Geometry: see drawing. Coordinates: mm, zero at the bounding-box minimum. A direction names the side the tool comes from. Coordinates: 2 decimals unless noted, no trailing zeros. Loops run counter-clockwise (first coordinate to the right, second up) from the corner with the lowest first, then second, coordinate; pieces in that order, holes last. Notation, with made-up numbers: (37.5, 20) -> (71.5, 20) arc R29 ccw to (71.5, 44) -> close; hole circle Ø3 at (86.25, -22). An arc over 180 degrees is marked (long way). Put each result on its own line as item: value. Start each with the question number.
1) Contact query for flat-ended pins moving along their axis: P1, Ø6, axis at x = 12, y = 6.5, coming from the +Z side; P2, Ø1.5, axis at x = 4, y = 2.5, coming from the -Z side. Output: stop coordinate, or through.
2) Cut plane D-D (y = 4.5). Return the cut outline in (x, z), plus the area to 3 significant figures.
3) Material intervals for L1, parallel to X at y = 9, z = 1.9; L2, parallel to X at y = 5, z = 2.7; L3, parallel to Y at x = 4, z = 2.35, sorted ascending.
4) Cut plane A-A (x = 4). Return the cut outline in (y, z).
5) Cut plane C-C (y = 9). Return the cut outline in (x, z).
6) Cut plane B-B (z = 2.35). Return the cut outline in (x, y), plus the area to 3 significant figures.
7) Set-up query: the marked faces 1 and 2. Return all of +Z, -Z, +X, -X, +Y, -Y with unobstructed straight access to the full face (end or side cutting, diameter ignored); none if empty.
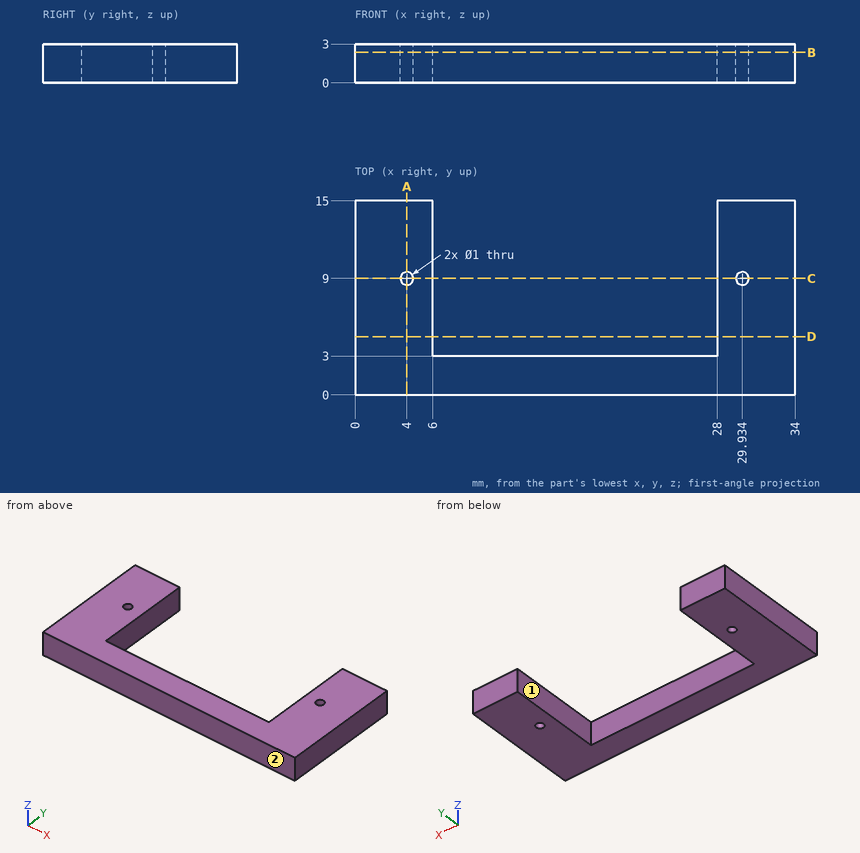
Results found:
1. P1: passes through
1. P2: stops at z = 0
2. outline: (0, 0) -> (6, 0) -> (6, 3) -> (0, 3) -> close; (28, 0) -> (34, 0) -> (34, 3) -> (28, 3) -> close
2. area: 36.0 mm2
3. L1: x = 0 to 3.5, 4.5 to 6, 28 to 29.43, 30.43 to 34
3. L2: x = 0 to 6, 28 to 34
3. L3: y = 0 to 8.5, 9.5 to 15
4. outline: (0, 0) -> (8.5, 0) -> (8.5, 3) -> (0, 3) -> close; (9.5, 0) -> (15, 0) -> (15, 3) -> (9.5, 3) -> close
5. outline: (0, 0) -> (3.5, 0) -> (3.5, 3) -> (0, 3) -> close; (4.5, 0) -> (6, 0) -> (6, 3) -> (4.5, 3) -> close; (28, 0) -> (29.43, 0) -> (29.43, 3) -> (28, 3) -> close; (30.43, 0) -> (34, 0) -> (34, 3) -> (30.43, 3) -> close
6. outline: (0, 0) -> (34, 0) -> (34, 15) -> (28, 15) -> (28, 3) -> (6, 3) -> (6, 15) -> (0, 15) -> close; hole circle Ø1 at (4, 9); hole circle Ø1 at (29.93, 9)
6. area: 244 mm2
7. face 1: +Z, -Z, +Y
7. face 2: +Z, -Z, +X, -X, -Y
